The listing builds one solid part. Answer for the finished solid, in the listing's coordinates (mm). Face numbers are marked on the shaded views. A direction names the side the tool comes from. Coordinates: 2 decimals unless noted, no trailing zeros. Order: outer loops, then holes, each group sorted by start corner. A loop starts at its lowest first (then second) coordinate and runs counter-clockwise, first axis right, second up. Notation, with made-up numbers: (-13.5, -6) -> (21.5, -6) arc R37 ccw to (21.5, 32) -> close; hole circle Ø8 at (85, 74). An arc over 180 degrees is marked (long way). Return JSON: item names as keys, results as strings.
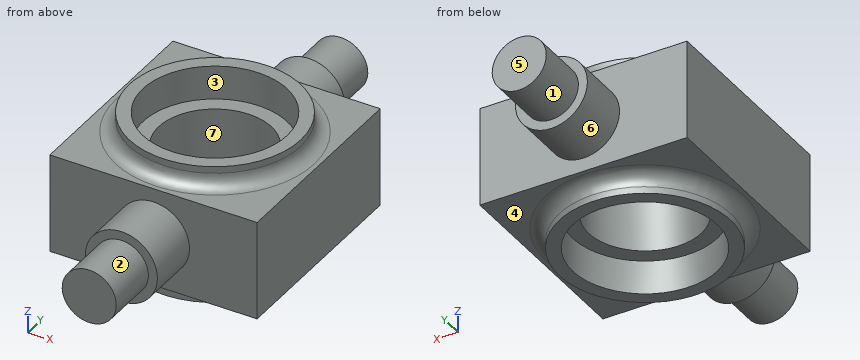
```python
from build123d import *

# Parameters (mm, degrees)
SKETCH1_W           = 46
SKETCH1_H           = 46
BOSS_EXTRUDE1_DEPTH = 11
SKETCH2_R           = 16
CUT_EXTRUDE1_DEPTH  = 3
SKETCH3_R           = 12.5
CUT_EXTRUDE2_DEPTH  = 38.669616404
SKETCH4_R           = 8
BOSS_EXTRUDE2_DEPTH = 12
SKETCH6_R           = 19
BOSS_EXTRUDE5_DEPTH = 4.5
SKETCH8_R           = 16
CUT_EXTRUDE6_DEPTH  = 7.5
FILLET1_R           = 3
SKETCH9_R           = 6
BOSS_EXTRUDE6_DEPTH = 12


with BuildPart() as part:
    # Sketch1 → Boss-Extrude1 (new, symmetric)
    with BuildSketch(Plane.XY):
        Rectangle(SKETCH1_W, SKETCH1_H)
    extrude(amount=BOSS_EXTRUDE1_DEPTH, both=True)

    # Sketch2 → Cut-Extrude1 (cut)
    with BuildSketch(Plane.XY.offset(11)):
        Circle(SKETCH2_R)
    extrude(amount=-CUT_EXTRUDE1_DEPTH, mode=Mode.SUBTRACT)

    # Sketch3 → Cut-Extrude2 (cut, through all)
    with BuildSketch(Plane.XY.offset(8)):
        Circle(SKETCH3_R)
    extrude(amount=-CUT_EXTRUDE2_DEPTH, mode=Mode.SUBTRACT)

    # Sketch4 → Boss-Extrude2 (add)
    with BuildSketch(Plane.XZ.offset(23)):
        with Locations(Location((0, 0, 0), (0, 0, 270))):
            Circle(SKETCH4_R)
    boss_extrude2 = extrude(amount=BOSS_EXTRUDE2_DEPTH)

    # Sketch6 → Boss-Extrude5 (add)
    with BuildSketch(Plane.XY.offset(11)):
        Circle(SKETCH6_R)
    boss_extrude5 = extrude(amount=BOSS_EXTRUDE5_DEPTH)

    # Sketch8 → Cut-Extrude6 (cut)
    with BuildSketch(Plane.XY.offset(15.5)):
        Circle(SKETCH8_R)
    cut_extrude6 = extrude(amount=-CUT_EXTRUDE6_DEPTH, mode=Mode.SUBTRACT)

    # Mirror2: Boss-Extrude5 across plane
    add(boss_extrude5.mirror(Plane.XY))

    # Mirror3: Cut-Extrude6 across plane
    add(cut_extrude6.mirror(Plane.XY), mode=Mode.SUBTRACT)

    # Fillet1
    fillet1_edges = [part.edges().sort_by_distance(p)[0] for p in [
        (-19, 0, 11),
        (-19, 0, -11),
    ]]
    fillet(fillet1_edges, radius=FILLET1_R)

    # Sketch9 → Boss-Extrude6 (add)
    with BuildSketch(Plane.XZ.offset(35)):
        with Locations(Location((0, 0, 0), (0, 0, 270))):
            Circle(SKETCH9_R)
    boss_extrude6 = extrude(amount=BOSS_EXTRUDE6_DEPTH)

    # Mirror4: Boss-Extrude2, Boss-Extrude6 across plane
    add(boss_extrude2.mirror(Plane.ZX))
    add(boss_extrude6.mirror(Plane.ZX))


solid = part.part
```
Item 1: Which of the six approach directions +Z, -Z, +X, -X, +Y, -Y give full straight-line access (tool end or side, diameter ignored) to the marked faces 1, 2, 3 and 4?
Answer list:
{"face 1": "+Y", "face 2": "-Y", "face 3": "+Z", "face 4": "-Z"}
Item 2: The part is cut by section C-C on z = 13. Determine the outline of the cut face in (x, y).
Answer list:
{"outline": "circle Ø38.34 at (0, 0); hole circle Ø32 at (0, 0)"}
Item 3: Find the intervals of material crossed by probe 1 along Y at (x, z) = (0, 10); probe 2 along Z at (x, y) = (13, 6.5); probe 3 along Y at (x, z) = (14.5, -2.5), in increasing order.
Answer list:
{"probe 1": "-23 to -16, 16 to 23", "probe 2": "-8 to 8", "probe 3": "-23 to 23"}
Item 4: Determine the mould class of the marked faces 5, 6 and 7 for opening direction X: pulls with the +X half, pulls with the -X half, needs draft (parallel to the pull), parting line crosses it, or undercut.
Answer list:
{"face 5": "needs draft", "face 6": "parting line crosses it", "face 7": "undercut"}
Item 5: The part is cut by section B-B on z = 0. Determine the outline of the cut face in (x, y), plus the area to 3 significant figures.
Answer list:
{"outline": "(-23, -23) -> (-8, -23) -> (-8, -35) -> (-6, -35) -> (-6, -47) -> (6, -47) -> (6, -35) -> (8, -35) -> (8, -23) -> (23, -23) -> (23, 23) -> (8, 23) -> (8, 35) -> (6, 35) -> (6, 47) -> (-6, 47) -> (-6, 35) -> (-8, 35) -> (-8, 23) -> (-23, 23) -> close; hole circle Ø25 at (0, 0)", "area": "2,300 mm2"}
Item 6: The part is cut by section A-A on y = 0. Determine the outline of the cut face in (x, z).
Answer list:
{"outline": "(-23, -11) -> (-22, -11) arc R3 cw to (-19, -14) -> (-19, -15.5) -> (-16, -15.5) -> (-16, -8) -> (-12.5, -8) -> (-12.5, 8) -> (-16, 8) -> (-16, 15.5) -> (-19, 15.5) -> (-19, 14) arc R3 cw to (-22, 11) -> (-23, 11) -> close; (12.5, -8) -> (16, -8) -> (16, -15.5) -> (19, -15.5) -> (19, -14) arc R3 cw to (22, -11) -> (23, -11) -> (23, 11) -> (22, 11) arc R3 cw to (19, 14) -> (19, 15.5) -> (16, 15.5) -> (16, 8) -> (12.5, 8) -> close"}
Item 7: Flat-ended cylindrical pins translate along their axes: pin 1 (23 mm diameter, centred on x = -3, y = -1, fed in from +Z); pin 2 (4 mm diameter, centred on x = -7.5, z = -3.5, fed in from +Y); pin 3 (1.5 mm diameter, centred on y = -27.5, z = 7.5, fed in from +X). Find the tip coordinate at first contact, or state that the pin passes through.
Answer list:
{"pin 1": "z = 8", "pin 2": "y = 35", "pin 3": "x = 4.29"}
